Input: part model. Units: mm. Frame: model coordinates. A direction names the side the tool comes from. Coordinates: 2 decimals unless noted, no trailing zeros. Write each loop counter-clockwise with the first axis right and the second up, starting at its lowest first coordinate (ties: lowest second). Pieces come first, ordered by that corner, then holes. Notation, with made-up numbers: M 19,80.25 L 50,80.25 A15 ccw 50,91.25 Z; hole C -18.5,81.5 d2. An arc over 180 degrees is marked long. Write each question's results on one line, items separated by ' | '. Start each with the question number.
1. Section query A-A, the plane y = 8.5. Output: boundary loops of the cut face in (x, z), and give its area (3 significant figures).
2. Set-up query: faces 5 (the flat face through (17, 5, 0)), 6 (the flat face through (18, 1.3, -8)), 7 (the flat face through (18, 4.5, -14)), 8 (the flat face through (17, 10, -14)), 9 (the flat face through (25, 5, -4)). Return all of +Z, -Z, +X, -X, +Y, -Y with unobstructed straight access to the full face (end or side cutting, diameter ignored); none if empty.
3. Section query D-D, the plane x = 20. Output: boundary loops of the cut face in (y, z).
4. Ray query, probe 1 along Z at (x, y) = (9.85, 7); probe 2 along X at (y, z) = (7.85, -23.5); probe 3 along Z at (x, y) = (16, 1.75). Return the intervals inside material, ascending.
5. First-contact query: pin 1 (1.5 mm diameter, centred on x = 24, z = -13.5, fed in from -Y); pin 2 (1.5 mm diameter, centred on x = 9.5, z = -23.5, fed in from +Y); pin 3 (0.5 mm diameter, centred on x = 21, z = -8.5, fed in from -Y). Flat tips, straight axial feed; report the tip coordinate or a pass-through.
6. Pull-direction query (Z, two-part tool) for faces 1 (the flat face through (34.7, 6, -13)), 2 (the flat face through (10, 5, -24)), 3 (the flat face through (17, 5, -27)), 4 (the cylindrical face through (24.655, 7.535, -24.987)); classes: +Z half, -Z half, draft (parallel to the pull), parting line (faces both ways), or undercut.
7. Section query B-B, the plane z = -3.5. Output: boundary loops of the cut face in (x, y), and give its area (3 significant figures).
8. Section query C-C, the plane x = 9.85. Output: boundary loops of the cut face in (y, z), and give its area (3 significant figures).
```python
from build123d import *

# Parameters (mm, degrees)
CROQUIS1_W              = 34.7
CROQUIS1_H              = 27
SALIENTE_EXTRUIR1_DEPTH = 10
CROQUIS2_R              = 1.5
CORTAR_EXTRUIR1_DEPTH   = 5
CORTAR_EXTRUIR2_DEPTH   = 34.7


with BuildPart() as part:
    # Croquis1 → Saliente-Extruir1 (new body)
    with BuildSketch(Plane(origin=(0, 0, 0), x_dir=(1, 0, 0), z_dir=(0, 1, 0))):
        with Locations((17.35, 13.5)):
            Rectangle(CROQUIS1_W, CROQUIS1_H)
    extrude(amount=SALIENTE_EXTRUIR1_DEPTH)

    # Croquis2 → Cortar-Extruir1 (cut)
    with BuildSketch(Plane(origin=(0, 10, 0), x_dir=(1, 0, 0), z_dir=(0, 1, 0))):
        with Locations((9.85, 23.5)):
            Circle(CROQUIS2_R)
        with Locations((24.849986467, 23.5)):
            Circle(CROQUIS2_R)
        with Locations((9.85, 3.5)):
            Circle(CROQUIS2_R)
        with Locations((24.849986467, 3.5)):
            Circle(CROQUIS2_R)
    extrude(amount=-CORTAR_EXTRUIR1_DEPTH, mode=Mode.SUBTRACT)

    # Croquis3 → Cortar-Extruir2 (cut)
    with BuildSketch(Plane(origin=(34.7, 0, 0), x_dir=(0, 0, -1), z_dir=(1, 0, 0))):
        Polygon((7.5, 0), (19.5, 0), (19.5, 1.3), (17.8, 1.3), (17.8, 3.1), (19.5, 3.1), (19.5, 4.5), (7.5, 4.5), (7.5, 3.1), (9.2, 3.1), (9.2, 1.3), (7.5, 1.3), align=None)
    extrude(amount=-CORTAR_EXTRUIR2_DEPTH, mode=Mode.SUBTRACT)


solid = part.part
```
Answer:
1) outline: M 0,-27 L 34.7,-27 L 34.7,0 L 0,0 Z; hole C 9.85,-23.5 d3; hole C 9.85,-3.5 d3; hole C 24.85,-23.5 d3; hole C 24.85,-3.5 d3 | area: 909 mm^2
2) face 5: +Z, +X, -X, +Y, -Y | face 6: +X, -X, -Y | face 7: +X, -X | face 8: +Z, -Z, +X, -X, +Y | face 9: +Y
3) outline: M 0,-27 L 10,-27 L 10,0 L 0,0 L 0,-7.5 L 1.3,-7.5 L 1.3,-9.2 L 3.1,-9.2 L 3.1,-7.5 L 4.5,-7.5 L 4.5,-19.5 L 3.1,-19.5 L 3.1,-17.8 L 1.3,-17.8 L 1.3,-19.5 L 0,-19.5 Z
4) probe 1: -27 to -25, -22 to -5, -2 to 0 | probe 2: 0 to 8.35, 11.35 to 23.35, 26.35 to 34.7 | probe 3: -27 to -17.8, -9.2 to 0
5) pin 1: y = 4.5 | pin 2: y = 5 | pin 3: y = 1.3
6) face 1: draft | face 2: undercut | face 3: -Z half | face 4: undercut
7) outline: M 0,0 L 34.7,0 L 34.7,10 L 26.35,10 L 26.35,5 L 23.35,5 L 23.35,10 L 11.35,10 L 11.35,5 L 8.35,5 L 8.35,10 L 0,10 Z | area: 317 mm^2
8) outline: M 0,-27 L 10,-27 L 10,-25 L 5,-25 L 5,-22 L 10,-22 L 10,-5 L 5,-5 L 5,-2 L 10,-2 L 10,0 L 0,0 L 0,-7.5 L 1.3,-7.5 L 1.3,-9.2 L 3.1,-9.2 L 3.1,-7.5 L 4.5,-7.5 L 4.5,-19.5 L 3.1,-19.5 L 3.1,-17.8 L 1.3,-17.8 L 1.3,-19.5 L 0,-19.5 Z | area: 192 mm^2
